```python
from build123d import *

# Parameters (mm, degrees)
SKETCH1_W           = 50
SKETCH1_H           = 32
BOSS_EXTRUDE1_DEPTH = 47.5
SKETCH5_W           = 50
SKETCH5_H           = 32
BOSS_EXTRUDE2_DEPTH = 60
SKETCH4_R           = 5
CUT_EXTRUDE1_DEPTH  = 75
CUT_EXTRUDE2_DEPTH  = 16.9


with BuildPart() as part:
    # Sketch1 → Boss-Extrude1 (new, symmetric)
    with BuildSketch(Plane(origin=(0, 0, 0), x_dir=(0, 0, -1), z_dir=(1, 0, 0))):
        Rectangle(SKETCH1_W, SKETCH1_H)
    extrude(amount=BOSS_EXTRUDE1_DEPTH, both=True)

    # Sketch3 → Cut-Revolve1 (revolve, cut)
    with BuildSketch(Plane(origin=(0, 0, 0), x_dir=(0, 0, -1), z_dir=(1, 0, 0))):
        Polygon((-25, -12.35), (-11.5, -12.35), (-11.5, -7.35), (11.5, -7.35), (11.5, -12.35), (25, -12.35), (25, 16.59588936), (-25, 16.59588936), align=None)
    revolve(axis=Axis((0, 17.65, -20.249126458), (0, 0, -1)), mode=Mode.SUBTRACT)

    # Sketch5 → Boss-Extrude2 (add)
    with BuildSketch(Plane(origin=(47.5, 0, 0), x_dir=(0, 0, -1), z_dir=(1, 0, 0))):
        Rectangle(SKETCH5_W, SKETCH5_H)
    extrude(amount=BOSS_EXTRUDE2_DEPTH)

    # Sketch4 → Cut-Extrude1 (cut)
    with BuildSketch(Plane(origin=(0, 16, 0), x_dir=(1, 0, 0), z_dir=(0, 1, 0))):
        with Locations(Location((-35, 0, 0), (0, 0, 270))):
            Circle(SKETCH4_R)
        with Locations(Location((35, 0, 0), (0, 0, 270))):
            Circle(SKETCH4_R)
        with Locations((77.75, -20.6)):
            Circle(SKETCH4_R)
        with Locations(Location((75.295878395, 1.01110333, 0), (0, 0, 270))):
            Circle(SKETCH4_R)
        with Locations((70.163995975, 23.188381743)):
            Circle(SKETCH4_R)
    extrude(amount=-CUT_EXTRUDE1_DEPTH, mode=Mode.SUBTRACT)

    # Sketch6 → Cut-Extrude2 (cut)
    with BuildSketch(Plane(origin=(0, 16, 0), x_dir=(1, 0, 0), z_dir=(0, 1, 0))):
        Polygon((97.41116956, -160.42016543), (40, 31.15), (103.809557411, 50.272921943), (161.220726971, -141.297243487), align=None)
    extrude(amount=-CUT_EXTRUDE2_DEPTH, mode=Mode.SUBTRACT)


solid = part.part
```
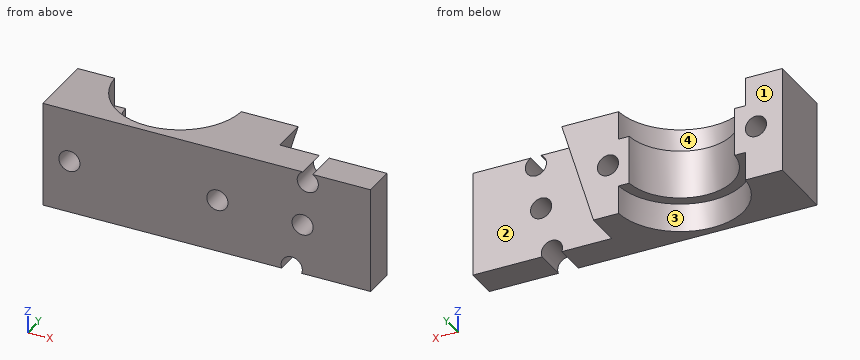
Input: part model. Units: mm. Frame: model coordinates. Face numbers are marked on the shaded views. A direction names the side the tool comes from. Coordinates: 2 decimals unless noted, no trailing zeros. Write each loop counter-clockwise with the first axis right and the second up, starting at its lowest first coordinate (ties: lowest second). Pieces come first, ordered by that corner, then holes. Notation, with made-up numbers: M 61,67 L 89,67 A16 cw 89,98 Z; hole C 86,89.25 d6. An arc over 180 degrees is marked long. Use one line per item in the form item = value.
Q1. Section D-D (y = -6). Return loops of the section in (x, z).
Answer below:
outline = M -47.5,-25 L -18.46,-25 L -18.46,-11.5 L -8.1,-11.5 L -8.1,11.5 L -18.46,11.5 L -18.46,25 L -47.5,25 Z; M 8.1,-11.5 L 18.46,-11.5 L 18.46,-25 L 65.5,-25 A5 cw long 74.82,-25 L 107.5,-25 L 107.5,25 L 80.12,25 A5 cw long 75.38,25 L 18.46,25 L 18.46,11.5 L 8.1,11.5 Z; hole C -35,0 d10; hole C 35,0 d10; hole C 75.3,-1.01 d10
Q2. Section A-A (y = 0.5). Return loops of the section in (x, z), plus the area to 3 significant figures.
Answer below:
outline = M -47.5,-25 L -24.61,-25 L -24.61,-11.5 L -18.19,-11.5 L -18.19,11.5 L -24.61,11.5 L -24.61,25 L -47.5,25 Z; M 18.19,-11.5 L 24.61,-11.5 L 24.61,-25 L 41.84,-25 L 56.83,25 L 24.61,25 L 24.61,11.5 L 18.19,11.5 Z; hole C -35,0 d10; hole C 35,0 d10
area = 2,520 mm²
Q3. First-contact query: pin 1 (5 mm diameter, centred on x = 3, z = -18, fed in from +Y); pin 2 (11.5 mm diameter, centred on x = 77.75, z = 20.6, fed in from +Y). Flat tips, straight axial feed; report the tip coordinate or a pass-through.
Answer below:
pin_1 = -11.84
pin_2 = -0.9
Q4. Material intervals for probe 1 along X at (y, z) = (-7, 20); probe 2 along X at (y, z) = (1, 0.5); probe 3 along X at (y, z) = (1, -16), sorted ascending. Write a range as from..to.
Answer below:
probe_1 = -47.5..-17.1, 17.1..72.79, 82.71..107.5
probe_2 = -47.5..-39.97, -30.03..-18.65, 18.65..30.03, 39.97..49.49
probe_3 = -47.5..-24.96, 24.96..44.54
Q5. Section B-B (x = -35). Return loops of the section in (y, z), plus the area to 3 significant figures.
Answer below:
outline = M -16,-25 L 16,-25 L 16,-5 L -16,-5 Z; M -16,5 L 16,5 L 16,25 L -16,25 Z
area = 1,280 mm²
Q6. Set-up query: the marked faces 1, 2, 3 and 4. Return all of +Z, -Z, +X, -X, +Y, -Y with unobstructed straight access to the full face (end or side cutting, diameter ignored); none if empty.
Answer below:
face_1 = +Z, -Z, +X, -X, +Y
face_2 = -Z, +X, +Y
face_3 = -Z, +Y
face_4 = +Z, +Y
Q7. Section C-C (z = 20.6). Return loops of the section in (x, y).
Answer below:
outline = M -47.5,-16 L 72.75,-16 L 72.75,-0.9 L 55.51,-0.9 L 55.51,16 L 29.95,16 A30 cw -29.95,16 L -47.5,16 Z; M 82.75,-16 L 107.5,-16 L 107.5,-0.9 L 82.75,-0.9 Z
